Autodesk Inventor part; units mm, degrees
ref_plane "YZ Plane" through (0, 0, 0) normal (1, 0, 0) x (0, 1, 0)
ref_plane "XZ Plane" through (0, 0, 0) normal (0, 1, 0) x (-1, 0, 0)
ref_plane "XY Plane" through (0, 0, 0) normal (0, 0, 1) x (1, 0, 0)
sketch "Szkic1" plane through (0, 0, 0) normal (0, 1, 0) x (-1, 0, 0)
  line L0 (12, 45) -> (0, 45)
  line L1 (0, 45) -> (0, -45)
  line L2 (0, -45) -> (12, -45)
  line L3 (12, -45) -> (12, 45)
  line L4 (0, 24) -> (-1.5, 24)
  line L5 (-1.5, 24) -> (-1.5, 6)
  line L6 (-1.5, 6) -> (0, 6)
  line L7 (0, 6) -> (0, 24)
  line L8 (0, -6) -> (-1.5, -6)
  line L9 (-1.5, -6) -> (-1.5, -24)
  line L10 (-1.5, -24) -> (0, -24)
  line L11 (0, -24) -> (0, -6)
  point P0 (0, 0)
  point P1 (0, -24)
  point P2 (0, 6)
  dimension "d0" = 90
  dimension "d1" = 12
  dimension "d2" = 45
  dimension "d3" = 21
  dimension "d4" = 18
  dimension "d5" = 1.5
  dimension "d6" = 21
  dimension "d7" = 18
extrude "Wyciągnięcie proste1" add sketch "Szkic1" along normal blind 39
sketch "Szkic2" plane through (-12, 0, -45) normal (-1, 0, 0) x (0, 0, 1)
  circle A0 centre (10, 32.5) radius 3.25
  circle A1 centre (10, 20.5) radius 3.25
  circle A2 centre (80, 32.5) radius 3.25
  circle A3 centre (80, 20.5) radius 3.25
  line L0 (0, 39) -> (90, 39)
  line L1 (0, 0) -> (0, 39)
  line L2 (90, 0) -> (90, 39)
  line L3 (0, 0) -> (20, 0)
  line L4 (20, 0) -> (20, 12)
  line L5 (20, 12) -> (0, 12)
  line L6 (0, 12) -> (0, 0)
  line L7 (0, 0) -> (90, 0)
  line L8 (90, 0) -> (70, 0)
  line L9 (70, 0) -> (70, 12)
  line L10 (70, 12) -> (90, 12)
  line L11 (90, 12) -> (90, 0)
  line L12 (13.0311, 37.75) -> (16.0622, 32.5)
  line L13 (16.0622, 32.5) -> (13.0311, 27.25)
  line L14 (13.0311, 27.25) -> (6.9689, 27.25)
  line L15 (6.9689, 27.25) -> (3.9378, 32.5)
  line L16 (3.9378, 32.5) -> (6.9689, 37.75)
  line L17 (6.9689, 37.75) -> (13.0311, 37.75)
  line L18 (13.0311, 25.75) -> (16.0622, 20.5)
  line L19 (16.0622, 20.5) -> (13.0311, 15.25)
  line L20 (13.0311, 15.25) -> (6.9689, 15.25)
  line L21 (6.9689, 15.25) -> (3.9378, 20.5)
  line L22 (3.9378, 20.5) -> (6.9689, 25.75)
  line L23 (6.9689, 25.75) -> (13.0311, 25.75)
  line L24 (76.9689, 25.75) -> (83.0311, 25.75)
  line L25 (83.0311, 25.75) -> (86.0622, 20.5)
  line L26 (86.0622, 20.5) -> (83.0311, 15.25)
  line L27 (83.0311, 15.25) -> (76.9689, 15.25)
  line L28 (76.9689, 15.25) -> (73.9378, 20.5)
  line L29 (73.9378, 20.5) -> (76.9689, 25.75)
  line L30 (76.9689, 37.75) -> (83.0311, 37.75)
  line L31 (83.0311, 37.75) -> (86.0622, 32.5)
  line L32 (86.0622, 32.5) -> (83.0311, 27.25)
  line L33 (83.0311, 27.25) -> (76.9689, 27.25)
  line L34 (76.9689, 27.25) -> (73.9378, 32.5)
  line L35 (73.9378, 32.5) -> (76.9689, 37.75)
  point P0 (45, 0)
  point P1 (0, 12)
  dimension "d10" = 6.5
  dimension "d11" = 6.5
  dimension "d12" = 10
  dimension "d13" = 12
  dimension "d14" = 10
  dimension "d15" = 20
  dimension "d16" = 12
  dimension "d17" = 20
  dimension "d18" = 10.5
  dimension "d19" = 10.5
  dimension "d20" = 10.5
  dimension "d21" = 10.5
extrude "Wyciągnięcie proste2" cut sketch "Szkic2" against normal through all contours A0 | A1 | A2 | A3 | L5 L4 L3 L1 | L2 L7 L9 L10
extrude "Wyciągnięcie proste3" cut sketch "Szkic2" against normal blind 6 contours A0 | A1 | A2 | A3 | L12 L13 L14 L15 L16 L17 | L18 L19 L20 L21 L22 L23 | L24 L25 L26 L27 L28 L29 | L30 L31 L32 L33 L34 L35
equation "\"d14\" = d12"
equation "\"d19\" = d18"
equation "\"d20\" = d18"
equation "\"d21\" = d18"
properties part number "YCarriageBackHolder" material "Tworzywo sztuczne ABS"
Read the model definition and answer for the solid it produces. Units are mm, in the model's axes. A direction names the side the tool comes from. Round coordinates to 2 decimals unless told otherwise and drop trailing zeros. Write each loop counter-clockwise with the first axis right and the second up, starting at its lowest first coordinate (ties: lowest second). Pieces come first, ordered by that corner, then holes.
Q1. Find section C-C on y = 13. Determine the outline of the cut face in (x, z).
Values:
outline: (-12, -45) - (0, -45) - (0, -24) - (1.5, -24) - (1.5, -6) - (0, -6) - (0, 6) - (1.5, 6) - (1.5, 24) - (0, 24) - (0, 45) - (-12, 45) - close
Q2. Find section A-A on x = -10.75. State how many separate pieces and enclosed holes the cut face has, and give its area (3 significant figures).
Values:
separate pieces: 1
enclosed holes: 4
area: 2,650 mm2
Q3. A tool of negligible diameter and unlimited length cuts with its end or side. For faces 1 (the face through (1, 19, -6)), 2 (the face through (1, 19, 24)), 3 (the face through (-6, 6, -25)), 4 (the face through (-6, 23, 38)), from which of +Z, -Z, +X, -X, +Y, -Y can it reach the whole face along a straight path? Write none if from no direction.
Values:
face 1: +X, +Y, -Y
face 2: +Z, +X, +Y, -Y
face 3: -Z, +X, -X, -Y
face 4: -X
Q4. Find section B-B on z = 35. Determine the outline of the cut face in (x, y).
Values:
outline: (-12, 12) - (0, 12) - (0, 17.25) - (-6, 17.25) - (-6, 15.25) - (-12, 15.25) - close; (-12, 25.75) - (-6, 25.75) - (-6, 23.75) - (0, 23.75) - (0, 29.25) - (-6, 29.25) - (-6, 27.25) - (-12, 27.25) - close; (-12, 37.75) - (-6, 37.75) - (-6, 35.75) - (0, 35.75) - (0, 39) - (-12, 39) - close
Q5. Flat-ended cylindrical pins translate along their axes: P1, Ø3, axis at y = 33.5, z = -32, coming from the -X side; P2, Ø3, axis at x = -8, z = -36, coming from the -Y side; P3, Ø6, axis at x = -4, y = 8.5, coming from the +Z side. Find the tip coordinate at first contact, or state that the pin passes through.
Values:
P1: stops at x = -6
P2: stops at y = 12
P3: stops at z = 25
Q6. Find section D-D on x = -3.25. Determine the outline of the cut face in (y, z).
Values:
outline: (0, -25) - (12, -25) - (12, -45) - (39, -45) - (39, 45) - (12, 45) - (12, 25) - (0, 25) - close; hole circle Ø6.5 at (20.5, -35); hole circle Ø6.5 at (20.5, 35); hole circle Ø6.5 at (32.5, -35); hole circle Ø6.5 at (32.5, 35)
Q7. Straight lines are drawn through the part: line 1 (Y direction, x = -3.9, z = -35); line 2 (Z direction, x = -10.75, y = 18); line 3 (Y direction, x = -2.5, z = 37). For each, find the intervals that lie inside material, in ascending order.
Values:
line 1: y = 12 to 17.25, 23.75 to 29.25, 35.75 to 39
line 2: z = -45 to -39.62, -30.38 to 30.38, 39.62 to 45
line 3: y = 12 to 17.94, 23.06 to 29.94, 35.06 to 39
Q8. The mould has two halves that part along Y. Classify faces 5 (the face through (-5, 39, 1)), 6 (the face through (-6, 25, 45)), 7 (the face through (-9.042, 17.912, 39.568)): released by +Y, released by -Y, zero draft, split by the parting line, or undercut.
Values:
face 5: released by +Y
face 6: zero draft
face 7: undercut
